from build123d import *

# Parameters (mm, degrees)
BOSS_EXTRUDE1_DEPTH = 1960
SKETCH2_R           = 25
BOSS_EXTRUDE2_DEPTH = 40
SKETCH3_W           = 1014.048392478
SKETCH3_H           = 10
CUT_EXTRUDE1_DEPTH  = 170


with BuildPart() as part:
    # Sketch1 → Boss-Extrude1 (new body)
    with BuildSketch(Plane(origin=(0, 0, 0), x_dir=(1, 0, 0), z_dir=(0, 1, 0))):
        with BuildLine():
            Line((300, -325), (300, 325))
            Line((300, 325), (-300, 325))
            Line((-300, 325), (-300, -325))
            ThreePointArc((-300, -325), (0, -345.183114428), (300, -325))
        make_face()
    extrude(amount=BOSS_EXTRUDE1_DEPTH)

    # Sketch2 → Boss-Extrude2 (add)
    with BuildSketch(Plane.XZ):
        with Locations((-247.421181531, 274.413092674)):
            Circle(SKETCH2_R)
        with Locations((247.421181531, 274.413092674)):
            Circle(SKETCH2_R)
        with Locations((247.421181531, -274.413092674)):
            Circle(SKETCH2_R)
        with Locations((-247.421181531, -274.413092674)):
            Circle(SKETCH2_R)
    extrude(amount=BOSS_EXTRUDE2_DEPTH)

    # Sketch3 → Cut-Extrude1 (cut)
    with BuildSketch(Plane(origin=(0, 0, 475), x_dir=(-1, 0, 0), z_dir=(0, 0, -1))):
        with Locations((0, 760)):
            Rectangle(SKETCH3_W, SKETCH3_H)
    extrude(amount=CUT_EXTRUDE1_DEPTH, mode=Mode.SUBTRACT)


solid = part.part
Input: part model. Units: mm. Frame: model coordinates. A direction names the side the tool comes from. Round coordinates to 2 decimals unless told otherwise and drop trailing zeros. Loops run counter-clockwise (first coordinate to the right, second up) from the corner with the lowest first, then second, coordinate; pieces in that order, holes last. Notation, with made-up numbers: (-12.5, 20) -> (37.5, 20) arc R16 ccw to (37.5, 34) -> close; hole circle Ø8 at (26, 25). An arc over 180 degrees is marked (long way). Answer as a JSON object with one key per item and string values. Group by question number.
1) Section query C-C on x = 124.5. Output: boundary loops of the cut face in (y, z), plus the area to 3 significant figures.
2) Draft query along X for faces 4 (the cylindrical face through (-4.21, 372.22, 345.18)), 5 (the cylindrical face through (-250.68, -19.72, 299.2)), 6 (the cylindrical face through (244.167, -19.72, -249.626)), 7 (the flat face through (-248, -40, 275)). Return one class per face: +X half, -X half, draft (parallel to the pull), parting line (faces both ways), or undercut.
3) Section query B-B on z = -41.5. Output: boundary loops of the cut face in (x, y).
4) Reachability of faces 1 (the flat face through (4, 765, 321)), 2 (the cylindrical face through (-250.676, -19.72, -249.626)), 3 (the cylindrical face through (-4.21, 1354.14, 345.18)) from +Z, -Z, +X, -X, +Y, -Y: full face, straight path, thin tool, end or side. Return the list, or none.
5) Pin query (flat end, axial travel): pin 1 (12 mm diameter, centred on x = -73.5, z = 320, fed in from -Y). Return the tip coordinate at first contact, or that it passes through.
6) Ray query, L1, parallel to Y at x = 70, z = 21; L2, parallel to Y at x = 54, z = 311; L3, parallel to Z at x = 28, y = 1486. Return the intervals inside material, ascending.
7) Section query A-A on x = -23. Output: boundary loops of the cut face in (y, z).
Reply:
{
 "1": {"outline": "(0, -325) -> (1960, -325) -> (1960, 341.72) -> (765, 341.72) -> (765, 305) -> (755, 305) -> (755, 341.72) -> (0, 341.72) -> close", "area": "1,310,000 mm2"},
 "2": {"face 4": "parting line", "face 5": "undercut", "face 6": "undercut", "face 7": "draft"},
 "3": {"outline": "(-300, 0) -> (300, 0) -> (300, 1960) -> (-300, 1960) -> close"},
 "4": {"face 1": "+Z, +X, -X", "face 2": "-Y", "face 3": "+Z, +Y, -Y"},
 "5": {"pin 1": "stops at y = 0"},
 "6": {"L1": "y = 0 to 1960", "L2": "y = 0 to 755, 765 to 1960", "L3": "z = -325 to 345.01"},
 "7": {"outline": "(0, -325) -> (1960, -325) -> (1960, 345.07) -> (765, 345.07) -> (765, 305) -> (755, 305) -> (755, 345.07) -> (0, 345.07) -> close"}
}
